from build123d import *

# Parameters (mm, degrees)
SKETCH1_W                = 275
SKETCH1_H                = 150
SKETCH1_R                = 5
BOSS_EXTRUDE1_DEPTH      = 20
SKETCH2_R                = 50
CUT_EXTRUDE1_DEPTH       = 169.769131064
SKETCH3_R                = 67.5
CUT_EXTRUDE2_DEPTH       = 10
SKETCH4_R                = 5
CUT_EXTRUDE3_DEPTH       = 169.769131064
SKETCH5_W                = 19.05
SKETCH5_H                = 6.48
CUT_EXTRUDE4_DEPTH       = 0.64
M2_CLEARANCE_HOLE1_D     = 2.6
M2_CLEARANCE_HOLE1_DEPTH = 2
M2_CLEARANCE_HOLE1_TIP   = 0.781118805


with BuildPart() as part:
    # Sketch1 → Boss-Extrude1 (new body)
    with BuildSketch(Plane(origin=(0, 0, 0), x_dir=(1, 0, 0), z_dir=(0, 1, 0))):
        with Locations((-12.36, 0)):
            Rectangle(SKETCH1_W, SKETCH1_H)
        with Locations(Location((0, 0, 0), (0, 0, 270))):
            Circle(SKETCH1_R, mode=Mode.SUBTRACT)
    extrude(amount=BOSS_EXTRUDE1_DEPTH)

    # Sketch2 → Cut-Extrude1 (cut, through all)
    with BuildSketch(Plane(origin=(0, 20, 0), x_dir=(1, 0, 0), z_dir=(0, 1, 0))):
        with Locations(Location((0, 0, 0), (0, 0, 270))):
            Circle(SKETCH2_R)
    extrude(amount=-CUT_EXTRUDE1_DEPTH, mode=Mode.SUBTRACT)

    # Sketch3 → Cut-Extrude2 (cut)
    with BuildSketch(Plane(origin=(0, 20, 0), x_dir=(1, 0, 0), z_dir=(0, 1, 0))):
        with Locations(Location((0, 0, 0), (0, 0, 270))):
            Circle(SKETCH3_R)
    extrude(amount=-CUT_EXTRUDE2_DEPTH, mode=Mode.SUBTRACT)

    # Sketch4 → Cut-Extrude3 (cut, through all)
    with BuildSketch(Plane(origin=(0, 20, 0), x_dir=(1, 0, 0), z_dir=(0, 1, 0))):
        with Locations(Location((100.14, 50, 0), (0, 0, 270))):
            Circle(SKETCH4_R)
        with Locations(Location((-124.86, 50, 0), (0, 0, 90))):
            Circle(SKETCH4_R)
    extrude(amount=-CUT_EXTRUDE3_DEPTH, mode=Mode.SUBTRACT)

    # Sketch5 → Cut-Extrude4 (cut)
    with BuildSketch(Plane.XZ):
        with Locations((-90.335, -71.76)):
            Rectangle(SKETCH5_W, SKETCH5_H)
        with Locations((65.615, -71.76)):
            Rectangle(SKETCH5_W, SKETCH5_H)
    extrude(amount=-CUT_EXTRUDE4_DEPTH, mode=Mode.SUBTRACT)

    # M2 Clearance Hole1
    with Locations(Plane(origin=(0, 0.64, 0), x_dir=(-1, 0, 0), z_dir=(0, -1, 0))):
        with Locations((95.9, 71.76), (84.77, 71.76), (-71.18, 71.76), (-60.20961626, 71.76)):
            Hole(M2_CLEARANCE_HOLE1_D / 2, depth=M2_CLEARANCE_HOLE1_DEPTH)
            with Locations((0, 0, -(M2_CLEARANCE_HOLE1_DEPTH + M2_CLEARANCE_HOLE1_TIP / 2))):  # 118° drill point
                Cone(0, M2_CLEARANCE_HOLE1_D / 2, M2_CLEARANCE_HOLE1_TIP, mode=Mode.SUBTRACT)


solid = part.part
Verification items for the finished model (mm, model axes). A direction names the side the tool comes from. Coordinates: 2 decimals unless noted, no trailing zeros. Order: outer loops, then holes, each group sorted by start corner. A loop starts at its lowest first (then second) coordinate and runs counter-clockwise, first axis right, second up.
1. Set-up check for faces 4 (the face through (15.02, 5.07, 47.69)), 5 (the face through (-90, 0.64, -72)), 6 (the face through (-59.884, 15.07, 31.147)): record each of +Z, -Z, +X, -X, +Y, -Y from which the full face is reachable in a straight line by a thin tool's end or side.
Results found:
face 4: +Y, -Y
face 5: -Z, -Y
face 6: +Y
2. Sectioned sample at B-B, the plane x = -124.86. Record the cut outline in (y, z).
Results found:
outline: (0, -75) - (20, -75) - (20, -55) - (0, -55) - close; (0, -45) - (20, -45) - (20, 75) - (0, 75) - close
3. Go/stop test with flat-tipped pins: pin 1 Ø3.5 at (x, z) = (-95.9, -71.76) entering from -Y; pin 2 Ø0.7 at (x, y) = (66, 0) entering from -Z; pin 3 Ø6 at (x, z) = (-124.86, -50) entering from +Y. Record where each tip stops, or that it passes through.
Results found:
pin 1: stops at y = 0.64
pin 2: stops at z = -68.52
pin 3: passes through
4. Sectioned sample at C-C, the plane y = 15.25. Record the cut outline in (x, z).
Results found:
outline: (-149.86, -75) - (125.14, -75) - (125.14, 75) - (-149.86, 75) - close; hole circle Ø10 at (-124.86, -50); hole circle Ø135 at (0, 0); hole circle Ø10 at (100.14, -50)
5. Scan lines: line 1 (X direction, y = 1.55, z = -71.76); line 2 (Z direction, x = -84.77, y = 1.75); line 3 (X direction, y = 8, z = -46). Record each from-to range of solid material in increasing order.
Results found:
line 1: x = -149.86 to -97.2, -94.6 to -86.07, -83.47 to 58.91, 61.51 to 69.88, 72.48 to 125.14
line 2: z = -75 to -73.06, -70.46 to 75
line 3: x = -149.86 to -127.86, -121.86 to -19.6, 19.6 to 97.14, 103.14 to 125.14
6. Sectioned sample at D-D, the plane z = -35. Record the cut outline in (x, y), and give its area (3 significant figures).
Results found:
outline: (-149.86, 0) - (-35.71, 0) - (-35.71, 10) - (-57.72, 10) - (-57.72, 20) - (-149.86, 20) - close; (35.71, 0) - (125.14, 0) - (125.14, 20) - (57.72, 20) - (57.72, 10) - (35.71, 10) - close
area: 3,630 mm2
7. Release check for a two-part mould opening along Z. For faces 1 (the face through (65, 0.64, -72)), 2 (the face through (0.3, 10, -50.3)), 3 (the face through (-14, 10, 75)) record: +Z half, -Z half, draft (parallel to the pull), parting line (faces both ways), or undercut.
Results found:
face 1: draft
face 2: undercut
face 3: +Z half
8. Sectioned sample at A-A, the plane z = 0. Record the cut outline in (x, y), and give its area (3 significant figures).
Results found:
outline: (-149.86, 0) - (-50, 0) - (-50, 10) - (-67.5, 10) - (-67.5, 20) - (-149.86, 20) - close; (50, 0) - (125.14, 0) - (125.14, 20) - (67.5, 20) - (67.5, 10) - (50, 10) - close
area: 3,150 mm2
